The drawing under review shows one solid part. Ordinate dimensions are in mm from its lowest x, y, z. A direction names the side the tool comes from. Give positions to 0.01 mm unless a question says otherwise; leave off trailing zeros. Order: outer loops, then holes, each group sorted by start corner. A loop starts at its lowest first (then second) coordinate and runs counter-clockwise, first axis right, second up. Notation, with made-up numbers: (25, 22) -> (69, 22) arc R31 ccw to (69, 54) -> close; hole circle Ø10 at (34, 12.25). An arc over 180 degrees is marked (long way). Use a Markdown table: item, result. Add a question column.
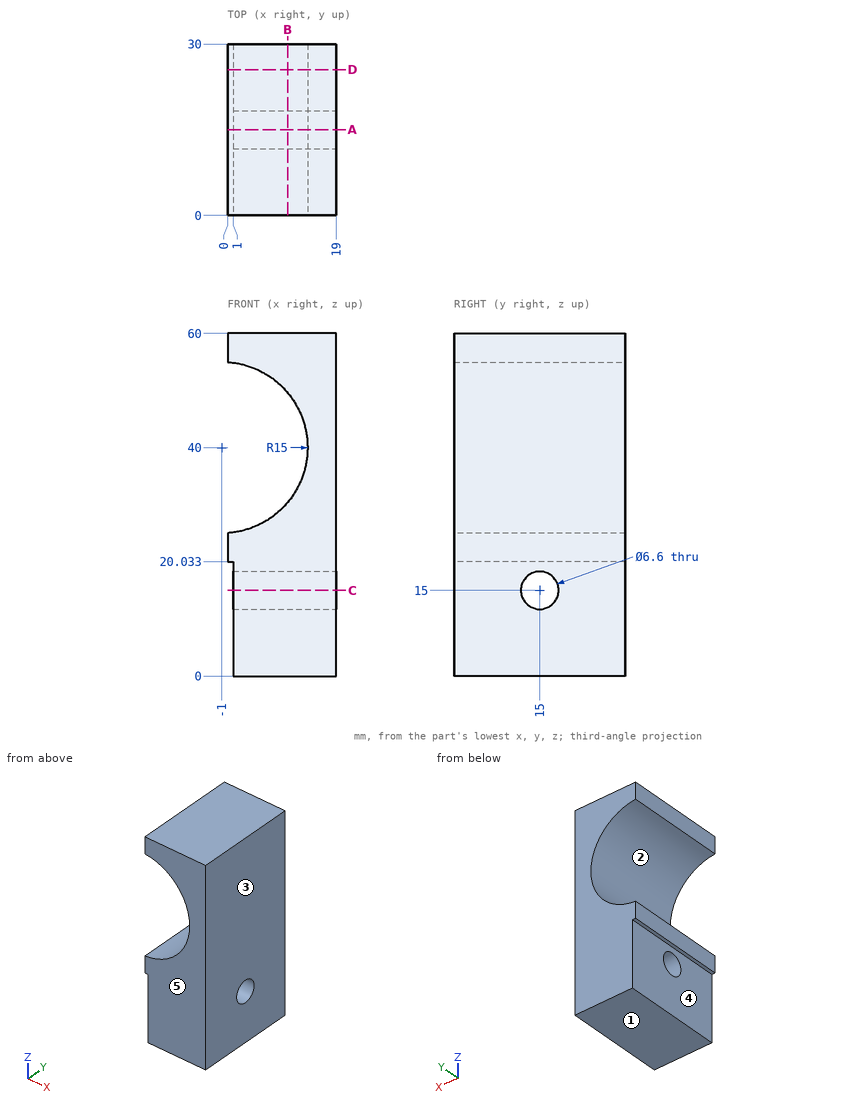
1) Machinability: for the marked faces 4 and 5, which of the approach directions +Z, -Z, +X, -X, +Y, -Y give a long, thin tool a straight path to every point of the face, cutting with its end or side? Answer none if there is none.
2) For L1, parallel to Z at x = 11, y = 15; L2, parallel to Y at x = 8.25, z = 15; L3, parallel to Z at x = 3.75, y = 13.75 (1 decimal), list the stretches that pass through material, from the lowest coordinate up. Write a range as [from, to].
3) Add section D-D (y = 25.5). Give the boundary of the cut face in (x, z).
4) Add section C-C (z = 15). Give the boundary of the cut face in (x, y), then the cut area to 3 significant figures.
5) Add section A-A (y = 15). Give the boundary of the cut face in (x, z).
6) Insertion check: pin 1 (16 mm diameter, centred on y = 12, z = 6.5, fed in from -X); pin 2 (8 mm diameter, centred on x = 3, y = 12, fed in from -Z); pin 3 (4 mm diameter, centred on y = 25.5, z = 45, fed in from -X). Each pin has a flat end and moves straight along its axis. Give the tip position at first contact, or say it passes through.
7) Add section B-B (x = 10.5). Give the boundary of the cut face in (y, z), then the cut area to 3 significant figures.
8) The part is to be moulded in two halves that separate along Z. For the marked faces 1, 2 and 3, say which applies: +Z half, -Z half, draft (parallel to the pull), parting line (faces both ways), or undercut.
Worked answers:
| question | item | result |
|---|---|---|
| 1 | face 4 | -Z, -X, +Y, -Y |
| 1 | face 5 | +Z, -Z, +X, -X, -Y |
| 2 | L1 | [0, 11.7], [18.3, 31], [49, 60] |
| 2 | L2 | [0, 11.7], [18.3, 30] |
| 2 | L3 | [0, 11.9], [18.1, 25.8], [54.2, 60] |
| 3 | outline | (0, 20.03) -> (1, 20.03) -> (1, 0) -> (19, 0) -> (19, 60) -> (0, 60) -> (0, 54.97) arc R15 cw to (0, 25.03) -> close |
| 4 | outline | (1, 0) -> (19, 0) -> (19, 11.7) -> (1, 11.7) -> close; (1, 18.3) -> (19, 18.3) -> (19, 30) -> (1, 30) -> close |
| 4 | area | 421 mm^2 |
| 5 | outline | (0, 20.03) -> (1, 20.03) -> (1, 18.3) -> (19, 18.3) -> (19, 60) -> (0, 60) -> (0, 54.97) arc R15 cw to (0, 25.03) -> close; (1, 0) -> (19, 0) -> (19, 11.7) -> (1, 11.7) -> close |
| 6 | pin 1 | x = 1 |
| 6 | pin 2 | z = 0 |
| 6 | pin 3 | x = 12.27 |
| 7 | outline | (0, 0) -> (30, 0) -> (30, 30.37) -> (0, 30.37) -> close; (0, 49.63) -> (30, 49.63) -> (30, 60) -> (0, 60) -> close; hole circle Ø6.6 at (15, 15) |
| 7 | area | 1,190 mm^2 |
| 8 | face 1 | -Z half |
| 8 | face 2 | undercut |
| 8 | face 3 | draft |
